```python
from build123d import *

# Parameters (mm, degrees)
SKETCH1_W            = 114.3
SKETCH1_H            = 203.2
BOSS_EXTRUDE1_DEPTH  = 6.35
CUT_EXTRUDE2_DEPTH   = 117.743329574
CUT_EXTRUDE3_DEPTH   = 117.743329574
CUT_EXTRUDE4_DEPTH   = 117.743329574
MIRROR3_COPY_1_DEPTH = 117.743329574
MIRROR3_COPY_2_DEPTH = 117.743329574
SKETCH7_R            = 1.651
CUT_EXTRUDE7_DEPTH   = 117.743329574
CUT_EXTRUDE8_DEPTH   = 117.743329574
LPATTERN1_COUNT      = 3
LPATTERN1_PITCH      = 19.05


with BuildPart() as part:
    # Sketch1 → Boss-Extrude1 (new body)
    with BuildSketch(Plane.XY):
        Rectangle(SKETCH1_W, SKETCH1_H)
    extrude(amount=BOSS_EXTRUDE1_DEPTH)

    # Sketch2 → Cut-Extrude2 (cut, through all)
    with BuildSketch(Plane.XY.offset(6.35)):
        Polygon((-57.15, 6.35), (-57.15, -6.35), (-50.8, -6.35), (-50.8, -1.651), (-45.72, -1.651), (-45.72, -3.81), (-42.926, -3.81), (-42.926, -1.651), (-39.116, -1.651), (-39.116, 1.651), (-42.926, 1.651), (-42.926, 3.81), (-45.72, 3.81), (-45.72, 1.651), (-50.8, 1.651), (-50.8, 6.35), align=None)
    cut_extrude2 = extrude(amount=-CUT_EXTRUDE2_DEPTH, mode=Mode.SUBTRACT)

    # Sketch3 → Cut-Extrude3 (cut, through all)
    with BuildSketch(Plane.XY.offset(6.35)):
        Polygon((-31.75, 101.6), (-31.75, 95.25), (-27.051, 95.25), (-27.051, 90.17), (-29.21, 90.17), (-29.21, 87.376), (-27.051, 87.376), (-27.051, 83.566), (-23.749, 83.566), (-23.749, 87.376), (-21.59, 87.376), (-21.59, 90.17), (-23.749, 90.17), (-23.749, 95.25), (-19.05, 95.25), (-19.05, 101.6), align=None)
    cut_extrude3 = extrude(amount=-CUT_EXTRUDE3_DEPTH, mode=Mode.SUBTRACT)

    # Sketch4 → Cut-Extrude4 (cut, through all)
    with BuildSketch(Plane.XY.offset(6.35)):
        Polygon((-57.15, 57.15), (-50.8, 57.15), (-50.8, 52.451), (-45.72, 52.451), (-45.72, 54.61), (-42.926, 54.61), (-42.926, 52.451), (-39.116, 52.451), (-39.116, 49.149), (-42.926, 49.149), (-42.926, 46.99), (-45.72, 46.99), (-45.72, 49.149), (-50.8, 49.149), (-50.8, 44.45), (-57.15, 44.45), align=None)
    cut_extrude4 = extrude(amount=-CUT_EXTRUDE4_DEPTH, mode=Mode.SUBTRACT)

    # Mirror1: Cut-Extrude3, Cut-Extrude4 across plane
    add(cut_extrude3.mirror(Plane.ZX), mode=Mode.SUBTRACT)
    add(cut_extrude4.mirror(Plane.ZX), mode=Mode.SUBTRACT)

    # Mirror3: Cut-Extrude2, Cut-Extrude3, Cut-Extrude4 across plane
    add(cut_extrude2.mirror(Plane(origin=(0, 0, 0), x_dir=(0, 0, 1), z_dir=(1, 0, 0))), mode=Mode.SUBTRACT)
    add(cut_extrude3.mirror(Plane(origin=(0, 0, 0), x_dir=(0, 0, 1), z_dir=(1, 0, 0))), mode=Mode.SUBTRACT)
    add(cut_extrude4.mirror(Plane(origin=(0, 0, 0), x_dir=(0, 0, 1), z_dir=(1, 0, 0))), mode=Mode.SUBTRACT)

    # Mirror3 copy 1 sketch → Mirror3 copy 1 (cut, through all)
    with BuildSketch(Plane(origin=(0, 0, 6.35), x_dir=(-1, 0, 0), z_dir=(0, 0, 1))):
        Polygon((-31.75, 101.6), (-31.75, 95.25), (-27.051, 95.25), (-27.051, 90.17), (-29.21, 90.17), (-29.21, 87.376), (-27.051, 87.376), (-27.051, 83.566), (-23.749, 83.566), (-23.749, 87.376), (-21.59, 87.376), (-21.59, 90.17), (-23.749, 90.17), (-23.749, 95.25), (-19.05, 95.25), (-19.05, 101.6), align=None)
    extrude(amount=-MIRROR3_COPY_1_DEPTH, mode=Mode.SUBTRACT)

    # Mirror3 copy 2 sketch → Mirror3 copy 2 (cut, through all)
    with BuildSketch(Plane(origin=(0, 0, 6.35), x_dir=(-1, 0, 0), z_dir=(0, 0, 1))):
        Polygon((-57.15, 57.15), (-50.8, 57.15), (-50.8, 52.451), (-45.72, 52.451), (-45.72, 54.61), (-42.926, 54.61), (-42.926, 52.451), (-39.116, 52.451), (-39.116, 49.149), (-42.926, 49.149), (-42.926, 46.99), (-45.72, 46.99), (-45.72, 49.149), (-50.8, 49.149), (-50.8, 44.45), (-57.15, 44.45), align=None)
    extrude(amount=-MIRROR3_COPY_2_DEPTH, mode=Mode.SUBTRACT)

    # Sketch7 → Cut-Extrude7 (cut, through all)
    with BuildSketch(Plane(origin=(0, 0, 0), x_dir=(-1, 0, 0), z_dir=(0, 0, -1))):
        with Locations((-44.45, 60.325)):
            Circle(SKETCH7_R)
        with Locations((44.45, 60.325)):
            Circle(SKETCH7_R)
        with Locations((44.45, -79.375)):
            Circle(SKETCH7_R)
        with Locations((-44.45, -79.375)):
            Circle(SKETCH7_R)
    extrude(amount=-CUT_EXTRUDE7_DEPTH, mode=Mode.SUBTRACT)

    # Sketch8 → Cut-Extrude8 (cut, through all)
    with BuildSketch(Plane.XY.offset(6.35)):
        with BuildLine():
            Line((26.9875, -76.98493382), (1.5875, -91.649630657))
            ThreePointArc((1.5875, -91.649630657), (0, -92.075), (-1.5875, -91.649630657))
            Line((-1.5875, -91.649630657), (-26.9875, -76.98493382))
            ThreePointArc((-26.9875, -76.98493382), (-28.149630657, -72.647803163), (-23.8125, -71.485672506))
            Line((-23.8125, -71.485672506), (0, -85.233825791))
            Line((0, -85.233825791), (23.8125, -71.485672506))
            ThreePointArc((23.8125, -71.485672506), (28.149630657, -72.647803163), (26.9875, -76.98493382))
        make_face()
    cut_extrude8 = extrude(amount=-CUT_EXTRUDE8_DEPTH, mode=Mode.SUBTRACT)

    # LPattern1: Cut-Extrude8 ×3
    with Locations(*[(0, i * LPATTERN1_PITCH, 0) for i in range(1, LPATTERN1_COUNT)]):
        add(cut_extrude8, mode=Mode.SUBTRACT)


solid = part.part
```
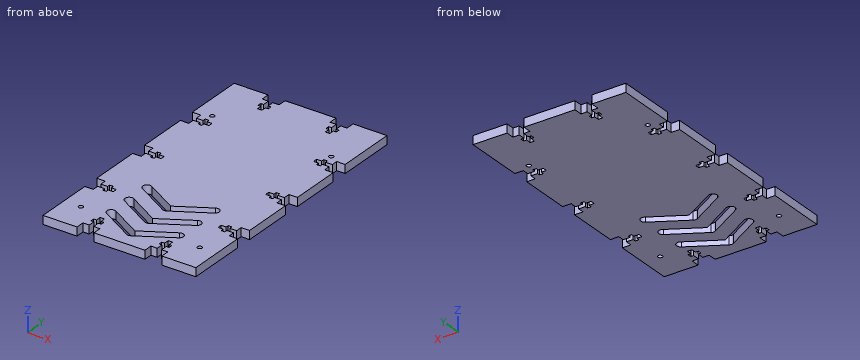
CAD build for the part. Positions are in the model's coordinates, mm. Give positions to 0.01 mm unless a question says otherwise; leave off trailing zeros. Order: outer loops, then holes, each group sorted by start corner. A loop starts at its lowest first (then second) coordinate and runs counter-clockwise, first axis right, second up.
(1) Saw through at B-B, the plane z = 2. State how many separate pieces and enclosed holes the cut face has, then the cut area to 3 significant figures.
(2) Flat gauge pins, fed straight in: pin 1 (2.5 mm diameter, centred on y = 46.5, z = 4.5, fed in from -X); pin 2 (1.7 mm diameter, centred on y = 2.5, z = 2.5, fed in from +X); pin 3 (1 mm diameter, centred on y = -51, z = 4.5, fed in from -X). Where does each tip first touch, or does it go through?
(3) Drill centre lines: L1, parallel to Y at x = -44.45, z = 5.25; L2, parallel to Y at x = 50.5, z = 3.5; L3, parallel to X at y = 85, z = 1. Where is each one in solid material? Low to high.
(4) Saw through at A-A, the plane y = -36.5. Give the cut face in (x, z).
Results found:
1. separate pieces: 1
1. enclosed holes: 7
1. area: 20,700 mm2
2. pin 1: stops at x = -50.8
2. pin 2: stops at x = 50.8
2. pin 3: stops at x = -39.12
3. L1: y = -101.6 to -81.03, -77.72 to -54.61, -46.99 to -3.81, 3.81 to 46.99, 54.61 to 58.67, 61.98 to 101.6
3. L2: y = -101.6 to -52.45, -49.15 to -1.65, 1.65 to 49.15, 52.45 to 101.6
3. L3: x = -57.15 to -27.05, -23.75 to 23.75, 27.05 to 57.15
4. outline: (-57.15, 0) - (-28.55, 0) - (-28.55, 6.35) - (-57.15, 6.35) - close; (-18.42, 0) - (18.42, 0) - (18.42, 6.35) - (-18.42, 6.35) - close; (28.55, 0) - (57.15, 0) - (57.15, 6.35) - (28.55, 6.35) - close
